Verification items for this drawing (mm, ordinates from the low corner). A direction names the side the tool comes from. Give positions to 0.01 mm unless a question says otherwise; leave off trailing zeros. Loops run counter-clockwise (first coordinate to the right, second up) from the corner with the lowest first, then second, coordinate; pieces in that order, holes last. Notation, with made-up numbers: (30, -9.75) -> (49, -9.75) arc R25 cw to (49, 26.25) -> close; hole circle Ø7 at (-10, -8). An arc over 180 degrees is marked (long way). Answer as a JSON object with one key per item and string values.
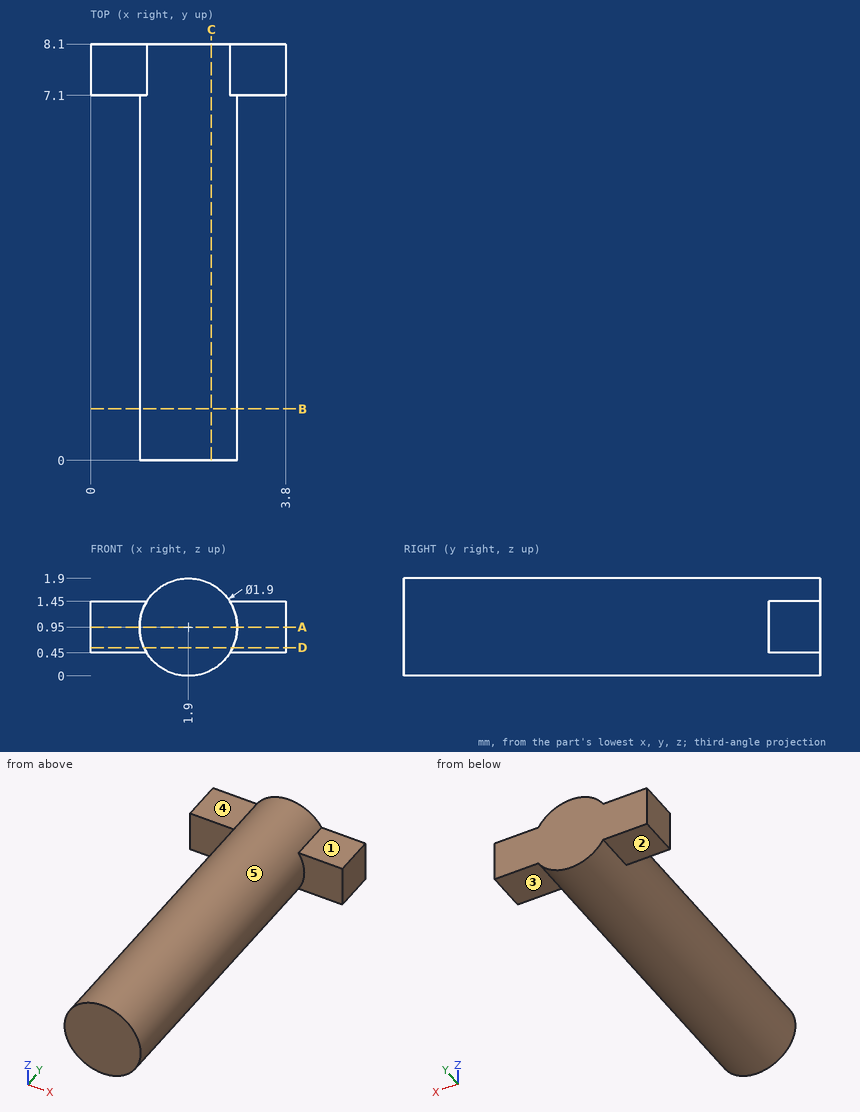
1) Section check C-C on x = 2.35. Record the cut outline in (y, z).
Geometry check:
{"outline": "(0, 0.11) -> (8.1, 0.11) -> (8.1, 1.79) -> (0, 1.79) -> close"}
2) Section check D-D on z = 0.55. Record the cut outline in (x, y).
Geometry check:
{"outline": "(0, 7.1) -> (1.04, 7.1) -> (1.04, 0) -> (2.76, 0) -> (2.76, 7.1) -> (3.8, 7.1) -> (3.8, 8.1) -> (0, 8.1) -> close"}
3) Section check A-A on z = 0.95. Record the cut outline in (x, y).
Geometry check:
{"outline": "(0, 7.1) -> (0.95, 7.1) -> (0.95, 0) -> (2.85, 0) -> (2.85, 7.1) -> (3.8, 7.1) -> (3.8, 8.1) -> (0, 8.1) -> close"}
4) Material ranges on line 1 along Y through (x, z) = (0.7, 1.25); line 2 along X through (y, z) = (3.25, 0.9); line 3 along Z through (x, y) = (1.95, 2.75), recorded low to high. Write a range as from..to.
Geometry check:
{"line 1": "y = 7.1..8.1", "line 2": "x = 0.95..2.85", "line 3": "z = 0..1.9"}
5) Section check B-B on y = 1. Record the cut outline in (x, z).
Geometry check:
{"outline": "circle Ø1.9 at (1.9, 0.95)"}
6) Tool access check on the marked faces 1, 2, 3, 4 and 5. Record the directions out of +Z, -Z, +X, -X, +Y, -Y that give a thin tool (end or side, any length) a straight path to the whole face; none if there is none.
Geometry check:
{"face 1": "+Z, +X, +Y, -Y", "face 2": "-Z, -X, +Y, -Y", "face 3": "-Z, +X, +Y, -Y", "face 4": "+Z, -X, +Y, -Y", "face 5": "-Y"}
7) Depth check by flat-ended pin: P1, Ø1.5, axis at x = 0.5, y = 2.5, coming from the +Z side; P2, Ø0.8, axis at x = 3.5, y = 7.5, coming from the -Z side; P3, Ø0.5, axis at x = 3.5, y = 7.5, coming from the +Z side. Enter the tip coordinate at first touch or a pass-through.
Geometry check:
{"P1": "stops at z = 1.64", "P2": "stops at z = 0.45", "P3": "stops at z = 1.45"}
